The listing builds one solid part. Answer for the finished solid, in the listing's coordinates (mm). Face numbers are marked on the shaded views. A direction names the side the tool comes from. Coordinates: 2 decimals unless noted, no trailing zeros. Write each loop counter-clockwise with the first axis right and the second up, starting at its lowest first coordinate (ties: lowest second). Pieces come first, ordered by that corner, then holes. Notation, with made-up numbers: M 28,38 L 62,38 A21 ccw 62,70 Z; hole C 48,37 d6. An arc over 180 degrees is marked long. Answer as CSV lines item,"result". Start each with the question number.
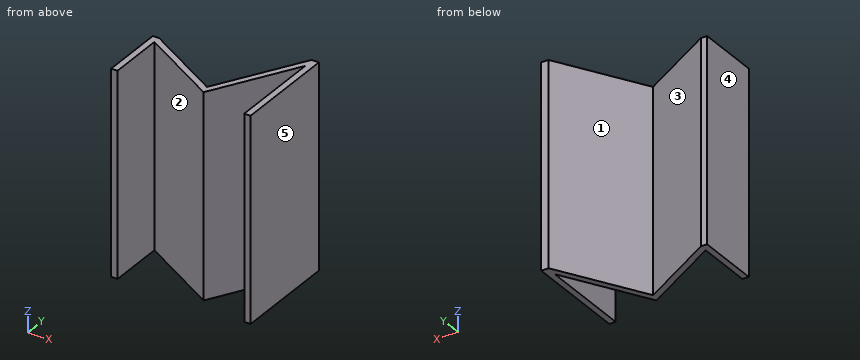
```python
from build123d import *

# Parameters (mm, degrees)
F1_DEPTH = 203.2


with BuildPart() as f1:
    # F0 (on Top) → F1 (new body)
    with BuildSketch(Plane.XY):
        Polygon((-97.927715, 63.5), (-97.927715, 0), (-91.577715, 0), (-91.577715, 56.167652), (-91.577715, 63.5), align=None)
        Polygon((-91.577715, 63.5), (-91.577715, 56.167652), (-12.263796, 10.375739), (35.361204, 92.864658), (35.361204, 0), (41.711204, 0), (41.711204, 103.863181), (34.378856, 103.863181), (-14.588057, 19.05), align=None)
    extrude(amount=F1_DEPTH)


solid = f1.part
```
1) Find the intervals of material crossed by line 1 (X direction, y = 45, z = 58); line 2 (X direction, y = 61, z = 51); line 3 (X direction, y = 28, z = 111), in increasing order. Write a range as from..to.
2) The part is cut by section C-C (y = 81). Determine the outline of the cut face in (x, z).
3) For a pull along X with two mould halves and no side action, classify the marked faces 3, 4 and 5 as +X half, -X half, draft (parallel to the pull), parting line (faces both ways), or undercut.
4) Which of the six approach directions +Z, -Z, +X, -X, +Y, -Y give full straight-line access (tool end or side, diameter ignored) to the marked faces 1 and 2?
5) The part is cut by section A-A (y = 58.5). Determine the outline of the cut face in (x, z), then the cut area to 3 significant figures.
6) Each of these flat-tipped pins is pushed along its axis until it touches: P1, Ø5, axis at y = 86.5, z = 24, coming from the -X side; P2, Ø1.5, axis at x = -50.5, z = 155.5, coming from the +Y side; P3, Ø5, axis at x = -94, z = 136, coming from the +Y side. Where does it stop, or does it pass through?
7) The part is cut by section B-B (z = 124). Determine the outline of the cut face in (x, y), then the cut area to 3 significant figures.
8) The part is cut by section D-D (x = -56.5). Determine the outline of the cut face in (y, z).
Completed:
1,line 1,"-97.93..-91.58, -72.23..-59.53, 0.39..7.73, 35.36..41.71"
1,line 2,"-97.93..-87.25, 9.63..16.96, 35.36..41.71"
1,line 3,"-97.93..-91.58, -42.79..-30.09, -9.42..-2.09, 35.36..41.71"
2,outline,"M 21.18,0 L 28.51,0 L 28.51,203.2 L 21.18,203.2 Z; M 35.36,0 L 41.71,0 L 41.71,203.2 L 35.36,203.2 Z"
3,face 3,"undercut"
3,face 4,"-X half"
3,face 5,"+X half"
4,face 1,"+Z, -Z, +Y"
4,face 2,"+Z, -Z, -Y"
5,outline,"M -97.93,0 L -82.92,0 L -82.92,203.2 L -97.93,203.2 Z; M 8.19,0 L 15.52,0 L 15.52,203.2 L 8.19,203.2 Z; M 35.36,0 L 41.71,0 L 41.71,203.2 L 35.36,203.2 Z"
5,area,"5,830 mm²"
6,P1,"x = 22.91"
6,P2,"y = 40.22"
6,P3,"y = 63.5"
7,outline,"M -97.93,0 L -91.58,0 L -91.58,56.17 L -12.26,10.38 L 35.36,92.86 L 35.36,0 L 41.71,0 L 41.71,103.86 L 34.38,103.86 L -14.59,19.05 L -91.58,63.5 L -97.93,63.5 Z"
7,area,"2,250 mm²"
8,outline,"M 35.92,0 L 43.25,0 L 43.25,203.2 L 35.92,203.2 Z"
